Answer from the drawing. Dimensions are ordinates in mm from the lowest x, y and z of the part. Give positions to 0.01 mm unless a question says otherwise; leave off trailing zeros. Write each loop counter-clockwise with the first axis right and the second up, starting at its lowest first coordinate (ties: lowest second). Pieces come first, ordered by that corner, then holes. Notation, with made-up numbers: M -7.5,-11.75 L 12.5,-11.75 A20 cw 12.5,0.25 Z; hole C 23.5,31.25 d9. An arc over 180 degrees is marked long. Answer as a JSON object with one key per item and string values.
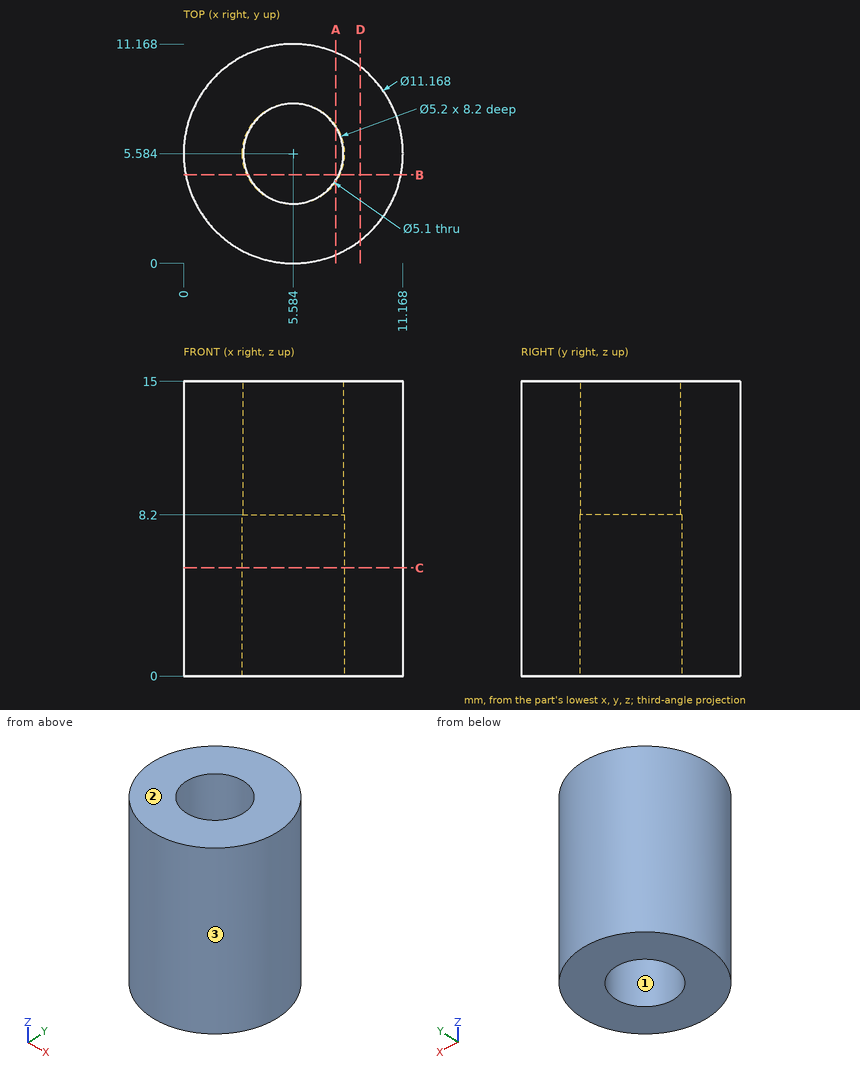
1. A cutting plane is placed at D-D, the plane x = 9. Give the vertices of the cut face in (y, z).
Verdict:
{"outline": "M 1.17,0 L 10,0 L 10,15 L 1.17,15 Z"}
2. A cutting plane is placed at A-A, the plane x = 7.75. Give the vertices of the cut face in (y, z), plus the area to 3 significant figures.
Verdict:
{"outline": "M 0.44,0 L 4.15,0 L 4.15,8.2 L 4.24,8.2 L 4.24,15 L 0.44,15 Z; M 6.93,8.2 L 7.02,8.2 L 7.02,0 L 10.73,0 L 10.73,15 L 6.93,15 Z", "area": "113 mm2"}
3. Consider line 1 along Y through (x, z) = (5.5, 1.5); line 2 along X through (y, z) = (7, 8.5); line 3 along Y through (x, z) = (4, 3). Determine where each line is inside the solid, lowest interval first.
Verdict:
{"line 1": "y = 0 to 2.99, 8.18 to 11.17", "line 2": "x = 0.18 to 3.46, 7.7 to 10.99", "line 3": "y = 0.23 to 3.52, 7.65 to 10.94"}
4. Flat-ended cylindrical pins translate along their axes: pin 1 (1 mm diameter, centred on x = 7.5, z = 8.5, fed in from -Y); pin 2 (3 mm diameter, centred on y = 2, z = 3.5, fed in from +X); pin 3 (3 mm diameter, centred on y = 1.5, z = 11, fed in from -X). Find the tip coordinate at first contact, or state that the pin passes through.
Verdict:
{"pin 1": "stops at y = 0.18", "pin 2": "stops at x = 10.76", "pin 3": "stops at x = 0.63"}
5. A cutting plane is placed at B-B, the plane y = 4.5. Give the vertices of the cut face in (x, z), plus the area to 3 significant figures.
Verdict:
{"outline": "M 0.11,0 L 3.22,0 L 3.22,8.2 L 3.28,8.2 L 3.28,15 L 0.11,15 Z; M 7.89,8.2 L 7.95,8.2 L 7.95,0 L 11.06,0 L 11.06,15 L 7.89,15 Z", "area": "94.2 mm2"}
6. The mould has two halves that part along X. Classify the marked faces 1, 2 and 3: released by +X, released by -X, zero draft, split by the parting line, or undercut.
Verdict:
{"face 1": "undercut", "face 2": "zero draft", "face 3": "split by the parting line"}
7. A cutting plane is placed at C-C, the plane z = 5.5. Give the vertices of the cut face in (x, y), plus the area to 3 significant figures.
Verdict:
{"outline": "C 5.58,5.58 d11.17; hole C 5.58,5.58 d5.2", "area": "76.7 mm2"}
